```python
from build123d import *

# Parameters (mm, degrees)
SKETCH1_R                = 250
SKETCH1_R_2              = 210.5
BOSS_EXTRUDE1_DEPTH      = 12.7
CUT_EXTRUDE1_DEPTH       = 354.781415566
FILLET1_R                = 1
CIRPATTERN1_COUNT        = 8
FILLET1_OF_CIRPATTERN1_R = 1
SKETCH6_W                = 40
SKETCH6_H                = 12.7
CUT_EXTRUDE4_DEPTH       = 354.665618911
SKETCH7_R                = 3.2
CUT_EXTRUDE5_DEPTH       = 354.665618911


with BuildPart() as part:
    # Sketch1 → Boss-Extrude1 (new body)
    with BuildSketch(Plane(origin=(0, 0, 0), x_dir=(1, 0, 0), z_dir=(0, 1, 0))):
        with Locations(Location((0, 0, 0), (0, 0, 270))):
            Circle(SKETCH1_R)
        with Locations(Location((0, 0, 0), (0, 0, 270))):
            Circle(SKETCH1_R_2, mode=Mode.SUBTRACT)
    extrude(amount=BOSS_EXTRUDE1_DEPTH)

    # Sketch2 → Cut-Extrude1 (cut, through all)
    with BuildSketch(Plane(origin=(0, 12.7, 0), x_dir=(1, 0, 0), z_dir=(0, 1, 0))):
        with BuildLine():
            Line((6.4, 225.5), (-6.4, 225.5))
            ThreePointArc((-6.4, 225.5), (-9.6, 228.7), (-6.4, 231.9))
            Line((-6.4, 231.9), (-6.4, 250))
            Line((-6.4, 250), (6.4, 250))
            Line((6.4, 250), (6.4, 231.9))
            ThreePointArc((6.4, 231.9), (9.6, 228.7), (6.4, 225.5))
        make_face()
    cut_extrude1 = extrude(amount=-CUT_EXTRUDE1_DEPTH, mode=Mode.SUBTRACT)

    # Fillet1
    fillet1_edges = [part.edges().sort_by_distance(p)[0] for p in [
        (-6.4, 6.35, -231.9),
        (6.4, 6.35, -231.9),
    ]]
    fillet(fillet1_edges, radius=FILLET1_R)

    # CirPattern1: Cut-Extrude1 ×8 about axis
    cirpattern1_axis = Axis((0, 0, 0), (0, 1, 0))
    for i in range(1, CIRPATTERN1_COUNT):
        add(cut_extrude1.rotate(cirpattern1_axis, i * 360 / CIRPATTERN1_COUNT), mode=Mode.SUBTRACT)

    # Fillet1 of CirPattern1
    fillet1_of_cirpattern1_edges = [part.edges().sort_by_distance(p)[0] for p in [
        (-168.503545957, 6.35, -159.452579158),
        (-159.452579158, 6.35, -168.503545957),
        (-231.9, 6.35, 6.4),
        (-231.9, 6.35, -6.4),
        (-159.452579158, 6.35, 168.503545957),
        (-168.503545957, 6.35, 159.452579158),
        (6.4, 6.35, 231.9),
        (-6.4, 6.35, 231.9),
        (168.503545957, 6.35, 159.452579158),
        (159.452579158, 6.35, 168.503545957),
        (231.9, 6.35, -6.4),
        (231.9, 6.35, 6.4),
        (159.452579158, 6.35, -168.503545957),
        (168.503545957, 6.35, -159.452579158),
    ]]
    fillet(fillet1_of_cirpattern1_edges, radius=FILLET1_OF_CIRPATTERN1_R)

    # Sketch6 → Cut-Extrude4 (cut, through all)
    with BuildSketch(Plane(origin=(0, 12.7, 0), x_dir=(1, 0, 0), z_dir=(0, 1, 0))):
        with Locations((-59.506660352, 216.85)):
            Rectangle(SKETCH6_W, SKETCH6_H)
        Polygon((-225.095552296, 92.887646728), (-221.442085646, 80.724498227), (-207.076162221, 85.039616318), (-210.72962887, 97.202764818), align=None)
    extrude(amount=-CUT_EXTRUDE4_DEPTH, mode=Mode.SUBTRACT)

    # Sketch7 → Cut-Extrude5 (cut, through all)
    with BuildSketch(Plane(origin=(0, 12.7, 0), x_dir=(1, 0, 0), z_dir=(0, 1, 0))):
        with Locations((-224.17499377, 89.822916397)):
            Circle(SKETCH7_R)
        with Locations((-218.377355315, 81.645056753)):
            Circle(SKETCH7_R)
        with Locations((-207.996720747, 88.104346648)):
            Circle(SKETCH7_R)
        with Locations((-213.794359201, 96.282206292)):
            Circle(SKETCH7_R)
        with Locations((-76.306660352, 223.2)):
            Circle(SKETCH7_R)
        with Locations((-42.706660352, 223.2)):
            Circle(SKETCH7_R)
        with Locations((-39.506660352, 213.7)):
            Circle(SKETCH7_R)
        with Locations((-76.306660352, 210.5)):
            Circle(SKETCH7_R)
    extrude(amount=-CUT_EXTRUDE5_DEPTH, mode=Mode.SUBTRACT)


solid = part.part
```
Verification items for the finished model (mm, model axes). A direction names the side the tool comes from. Round coordinates to 2 decimals unless told otherwise and drop trailing zeros. Write each loop counter-clockwise with the first axis right and the second up, starting at its lowest first coordinate (ties: lowest second). Pieces come first, ordered by that corner, then holes. Notation, with made-up numbers: (43.5, 23.25) -> (61.5, 23.25) arc R21 ccw to (61.5, 54.25) -> close; hole circle Ø2 at (8, -31). An arc over 180 degrees is marked (long way). Write each question's results on one line, items separated by ' | '.
Q1. Sectioned sample at A-A, the plane z = 0. Record the boundary of the cut face in (x, y), and give its area (3 significant figures).
Derived:
outline: (-225.5, 0) -> (-210.5, 0) -> (-210.5, 12.7) -> (-225.5, 12.7) -> close; (210.5, 0) -> (225.5, 0) -> (225.5, 12.7) -> (210.5, 12.7) -> close | area: 381 mm²
Q2. Sectioned sample at D-D, the plane y = 6.5. Give the number of separate pieces and of enclosed holes in the cut face, and give its area (3 significant figures).
Derived:
separate pieces: 1 | enclosed holes: 3 | area: 53,600 mm²
Q3. Sectioned sample at C-C, the plane x = -54.5. Record the boundary of the cut face in (y, z).
Derived:
outline: (0, -243.99) -> (12.7, -243.99) -> (12.7, -223.2) -> (0, -223.2) -> close; (0, -210.5) -> (12.7, -210.5) -> (12.7, -203.32) -> (0, -203.32) -> close; (0, 203.32) -> (12.7, 203.32) -> (12.7, 243.99) -> (0, 243.99) -> close
Q4. Sectioned sample at B-B, the plane x = 78.5. Record the boundary of the cut face in (y, z), and give its area (3 significant figures).
Derived:
outline: (0, -237.36) -> (12.7, -237.36) -> (12.7, -195.32) -> (0, -195.32) -> close; (0, 195.32) -> (12.7, 195.32) -> (12.7, 237.36) -> (0, 237.36) -> close | area: 1,070 mm²
Q5. Go/stop test with flat-tipped pins: pin 1 Ø6.5 at (y, z) = (4.5, -2.5) entering from +X; pin 2 Ø6 at (x, y) = (-95.5, 4.5) entering from +Z; pin 3 Ø6 at (y, z) = (6.5, -85.5) entering from -X. Record where each tip stops, or that it passes through.
Derived:
pin 1: stops at x = 225.5 | pin 2: stops at z = 232.26 | pin 3: stops at x = -236
Q6. Thickness scan on probe 1 along Z at (x, y) = (-168.5, 11.25); probe 2 along Z at (x, y) = (-158.5, 1); probe 3 along X at (y, z) = (5.25, 0). Record the ranges inside material, lowest first.
Derived:
probe 1: z = -184.68 to -177.55, -154.92 to -126.17, 126.17 to 154.92, 177.55 to 184.68 | probe 2: z = -193.33 to -169.16, -160.41 to -138.52, 138.52 to 160.41, 169.16 to 193.33 | probe 3: x = -225.5 to -210.5, 210.5 to 225.5
Q7. Access from +Z, -Z, +X, -X, +Y, -Y to the whole of each face (thin tool, end or side, straight path). Record for faces 1 (the face through (-60, 6, -223.2)), 2 (the face through (241, 6, -6.4)), 3 (the face through (-241, 6, 6.4)), 4 (the face through (0, 6, -225.5)).
Derived:
face 1: +Y, -Y | face 2: +X, +Y, -Y | face 3: -X, +Y, -Y | face 4: -Z, +Y, -Y
Q8. Draft check along Z on faces 5 (the face through (-175.27, 6.44, 166.22)), 6 (the face through (94.48, 6.26, 231.46)), 7 (the face through (-230.475, 6.261, -96.857)). Enter one of: released by +Z, released by -Z, zero draft, split by the parting line, or undercut.
Derived:
face 5: undercut | face 6: released by +Z | face 7: released by -Z
